For this review, take the finished solid that the model builds, in its own axes (mm). A direction names the side the tool comes from. Give positions to 0.01 mm unless a question says otherwise; leave off trailing zeros. Order: outer loops, then holes, each group sorted by start corner. A loop starts at its lowest first (then second) coordinate and runs counter-clockwise, first axis right, second up. Notation, with made-up numbers: M 36.5,-16 L 95.5,-16 A23 ccw 95.5,0 Z; hole C 37.25,18 d6. An arc over 180 degrees is marked long. Use CSV: the item, a comma, the result in double quotes. Start each with the question number.
(1) Consider section D-D (x = -2). Write out the cut boundary in (y, z).
(2) Clearance check with flat-ended pins moving along their axes: P1, Ø2, axis at x = -3, y = 2, coming from the -Z side; P2, Ø2, axis at x = -49.5, y = 2.5, coming from the -Z side; P3, Ø2, axis at y = 2, z = -5.5, coming from the -X side; P4, Ø2, axis at x = -28.5, z = 6.5, coming from the -Y side. State where each tip first meets the part, or that it passes through.
(3) Wall thickness on L1, parallel to Z at x = 10.5, y = 0.75; L2, parallel to X at y = 3, z = 20.5; L3, parallel to X at y = 0.5, z = 36: over which ranges is each line inside the solid? List them lowest first. Write a range as from..to.
(4) Consider section B-B (z = 55). Write out the cut boundary in (x, y).
(5) Consider section A-A (x = 14). Write out the cut boundary in (y, z), and give its area (3 significant figures).
(6) Consider section C-C (z = 37). Write out the cut boundary in (x, y), and give its area (3 significant figures).
(7) Draft analysis for pull direction Z (two halves, no side actions). For faces 1 (the face through (12.931, 3.402, -53.897)), 2 (the face through (0, 3, 51.404)), 3 (the face through (-1, 0, -1)), state which applies: pulls with the +Z half, pulls with the -Z half, needs draft (parallel to the pull), parting line crosses it, or undercut.
(8) Tool access review of faces 4 (the face through (-12.82, 3.4, 63.97)), 5 (the face through (53, 3, -15.75)), 6 (the face through (-46.885, 3.498, -36.595)), 7 (the face through (-22.55, 3.4, 38.61)), 8 (the face through (8.25, 3, -59)): name each direction out of +Z, -Z, +X, -X, +Y, -Y from which nothing blocks a thin tool from reaching the whole face with its end or side.
```python
from build123d import *

# Parameters (mm, degrees)
BOSS_EXTRUDE3_DEPTH = 6.9
CUT_EXTRUDE1_DEPTH  = 10


with BuildPart() as part:
    # Sketch10 → Boss-Extrude3 (new body)
    with BuildSketch(Plane(origin=(0, 0, 0), x_dir=(1, 0, 0), z_dir=(0, 1, 0))):
        Polygon((-44.545662223, 45.655350227), (-61.811524227, 35.686900152), (-61.811524227, 15.75), (-44.711524227, 15.75), (-44.711524227, -15.75), (-61.811524227, -15.75), (-61.811524227, -35.686900152), (-44.545662223, -45.655350227), (-35.995662223, -30.846315823), (-8.715862004, -46.596315823), (-17.265862004, -61.405350227), (0, -71.373800303), (17.265862004, -61.405350227), (8.715862004, -46.596315823), (35.995662223, -30.846315823), (44.545662223, -45.655350227), (61.811524227, -35.686900152), (61.811524227, -15.75), (44.711524227, -15.75), (44.711524227, 15.75), (61.811524227, 15.75), (61.811524227, 35.686900152), (44.545662223, 45.655350227), (35.995662223, 30.846315823), (8.715862004, 46.596315823), (17.265862004, 61.405350227), (0, 71.373800303), (-17.265862004, 61.405350227), (-8.715862004, 46.596315823), (-35.995662223, 30.846315823), align=None)
    extrude(amount=BOSS_EXTRUDE3_DEPTH)

    # Sketch11 → Cut-Extrude1 (cut)
    with BuildSketch(Plane(origin=(0, 6.9, 0), x_dir=(1, 0, 0), z_dir=(0, 1, 0))):
        Polygon((-40.392179181, 32.846714965), (-53.561524227, 40.450039872), (-61.811524227, 35.686900152), (-61.811524227, 26.16062071), (-48.642179181, 18.557295803), align=None)
        Polygon((0, 71.373800303), (-8.25, 66.610660582), (-8.25, 51.404010768), (8.25, 51.404010768), (8.25, 66.610660582), align=None)
        Polygon((61.811524227, 35.686900152), (53.561524227, 40.450039872), (40.392179181, 32.846714965), (48.642179181, 18.557295803), (61.811524227, 26.16062071), align=None)
        Polygon((61.811524227, -35.686900152), (61.811524227, -26.16062071), (48.642179181, -18.557295803), (40.392179181, -32.846714965), (53.561524227, -40.450039872), align=None)
        Polygon((-8.25, -51.404010768), (-8.25, -66.610660582), (0, -71.373800303), (8.25, -66.610660582), (8.25, -51.404010768), align=None)
        Polygon((-48.642179181, -18.557295803), (-61.811524227, -26.16062071), (-61.811524227, -35.686900152), (-53.561524227, -40.450039872), (-40.392179181, -32.846714965), align=None)
    extrude(amount=-CUT_EXTRUDE1_DEPTH, mode=Mode.SUBTRACT)


solid = part.part
```
Check result:
1,outline,"M 0,-51.4 L 6.9,-51.4 L 6.9,51.4 L 0,51.4 Z"
2,P1,"stops at z = -51.4"
2,P2,"stops at z = -43.37"
2,P3,"stops at x = -44.71"
2,P4,"stops at y = 0"
3,L1,"z = -65.31..-49.69, -45.57..45.57, 49.69..65.31"
3,L2,"x = -61.81..-52.01, -47.52..47.52, 52.01..61.81"
3,L3,"x = -45.85..-38.97, -27.07..27.07, 38.97..45.85"
4,outline,"M -13.57,0 L -8.25,0 L -8.25,6.9 L -13.57,6.9 Z; M 8.25,0 L 13.57,0 L 13.57,6.9 L 8.25,6.9 Z"
5,outline,"M 0,-63.29 L 6.9,-63.29 L 6.9,-55.75 L 0,-55.75 Z; M 0,-43.55 L 6.9,-43.55 L 6.9,43.55 L 0,43.55 Z; M 0,55.75 L 6.9,55.75 L 6.9,63.29 L 0,63.29 Z"
5,area,"705 mm^2"
6,outline,"M -47.59,0 L -39.55,0 L -39.55,6.9 L -47.59,6.9 Z; M -25.34,0 L 25.34,0 L 25.34,6.9 L -25.34,6.9 Z; M 39.55,0 L 47.59,0 L 47.59,6.9 L 39.55,6.9 Z"
6,area,"461 mm^2"
7,face 1,"undercut"
7,face 2,"pulls with the +Z half"
7,face 3,"needs draft"
8,face 4,"+Z, -X, +Y, -Y"
8,face 5,"+X, +Y, -Y"
8,face 6,"-X, +Y, -Y"
8,face 7,"+Y, -Y"
8,face 8,"-Z, +Y, -Y"
